```python
from build123d import *

# Parameters (mm, degrees)
PAD_DEPTH       = 50
POCKET_DEPTH    = 50.001
FILLET_R        = 0.5
SKETCH003_R     = 7.438429
POCKET001_DEPTH = 24.66558


with BuildPart() as part:
    # Sketch → Pad (new body)
    with BuildSketch(Plane.XY):
        with BuildLine():
            Line((0, 15), (0, 0))
            Line((0, 0), (50, 0))
            Line((50, 0), (50, 20))
            ThreePointArc((50, 20), (47.363119, 25.733162), (41.294118, 27.462185))
            Line((41.294118, 27.462185), (6, 22))
            ThreePointArc((6, 22), (1.705266, 19.609772), (0, 15))
        make_face()
    extrude(amount=PAD_DEPTH)

    # Sketch002 → Pocket (cut, through all)
    with BuildSketch(Plane.XY):
        with BuildLine():
            Line((1.617649, 14.859023), (1.617649, 2.886441))
            Line((1.617649, 2.886441), (48.358659, 2.886441))
            Line((48.358659, 2.886441), (48.358659, 20.203976))
            ThreePointArc((48.358659, 20.203976), (46.261778, 24.757846), (41.4384, 26.125203))
            Line((41.4384, 26.125203), (6.589663, 20.669917))
            ThreePointArc((6.589663, 20.669917), (3.030296, 18.682876), (1.617649, 14.859023))
        make_face()
    extrude(amount=POCKET_DEPTH, mode=Mode.SUBTRACT)

    # Fillet
    fillet_edges = [part.edges().sort_by_distance(p)[0] for p in [
        (25, 0, 50),
        (0, 7.5, 50),
        (1.705266, 19.609772, 50),
        (23.647059, 24.731092, 50),
        (47.363119, 25.733162, 50),
        (50, 10, 50),
        (50, 10, 0),
        (25, 0, 0),
        (50, 0, 25),
        (0, 0, 25),
    ]]
    fillet(fillet_edges, radius=FILLET_R)

    # Sketch003 (on Face21 of Fillet) → Pocket001 (cut, through all)
    with BuildSketch(Plane(origin=(0, 2.886441, 0), x_dir=(-1, 0, 0), z_dir=(0, 1, 0))):
        with Locations((-24.985147, 24.818342)):
            Circle(SKETCH003_R)
    extrude(amount=POCKET001_DEPTH, mode=Mode.SUBTRACT)


solid = part.part
```
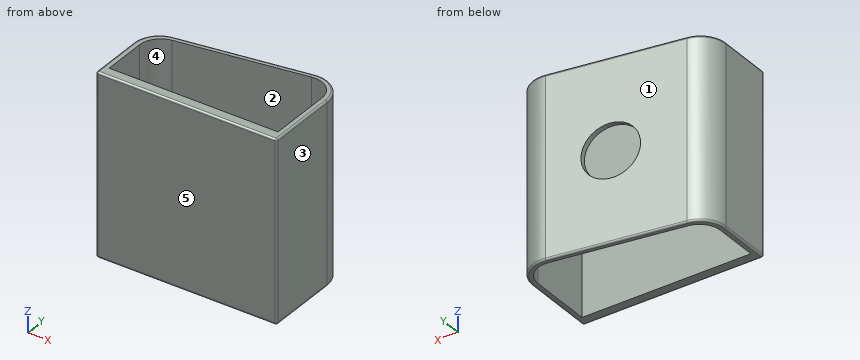
Can you work these out from the model? Positions are in its coordinate system, mm. Face numbers are marked on the shaded views. A direction names the side the tool comes from. Round coordinates to 2 decimals unless told otherwise and drop trailing zeros. Loops run counter-clockwise (first coordinate to the right, second up) from the corner with the lowest first, then second, coordinate; pieces in that order, holes last. Notation, with made-up numbers: M 3.25,7 L 38.25,7 A16 ccw 38.25,37 Z; hole C 29.25,-15 d4. An arc over 180 degrees is marked long. Answer in a Markdown table with one row per item.
1. If we section it at A-A, the plane y = 13.75: Please give me the cut outline in (x, z), plus the area to 3 significant figures.
Established:
| item | result |
|---|---|
| outline | M 0,0.5 A0.5 ccw 0.5,0 L 1.62,0 L 1.62,50 L 0.5,50 A0.5 ccw 0,49.5 Z; M 48.36,0 L 49.5,0 A0.5 ccw 50,0.5 L 50,49.5 A0.5 ccw 49.5,50 L 48.36,50 Z |
| area | 163 mm² |
2. If we section it at D-D, the plane x = 28: Give the number of separate pieces and of enclosed holes in the cut face, plus the area to 3 significant figures.
Established:
| item | result |
|---|---|
| separate pieces | 3 |
| enclosed holes | 0 |
| area | 194 mm² |
3. If we section it at C-C, the plane z = 27: Please give me the cut outline in (x, y).
Established:
| item | result |
|---|---|
| outline | M 0,0.5 A0.5 ccw 0.5,0 L 49.5,0 A0.5 ccw 50,0.5 L 50,20 A7.55 ccw 41.29,27.46 L 32.1,26.04 L 32.1,24.66 L 41.44,26.13 A5.99 cw 48.36,20.2 L 48.36,2.89 L 1.62,2.89 L 1.62,14.86 A5.88 cw 6.59,20.67 L 17.87,22.44 L 17.87,23.84 L 6,22 A7.08 ccw 0,15 Z |
4. On a 3-axis mill with a long thin cutter (end or side, diameter ignored), from which of +Z, -Z, +X, -X, +Y, -Y can I reach the whole of each face in a straight line? I mean the marked faces 4 and 5. Say none if no direction works.
Established:
| item | result |
|---|---|
| face 4 | +Z, -Z |
| face 5 | +Z, -Z, +X, -X, -Y |
5. Please list where these lines run through material, in increasing order: line 1 (X direction, y = 12.5, z = 34); line 2 (Y direction, x = 26.5, z = 29.5); line 3 (Y direction, x = 32, z = 19). Write a range as from..to.
Established:
| item | result |
|---|---|
| line 1 | 0..1.62, 48.36..50 |
| line 2 | 0..2.89 |
| line 3 | 0..2.89, 24.65..26.02 |
6. I'm going to push flat-ended pins straight in: pin 1 Ø5 at (x, z) = (18, 25.5) entering from +Y; pin 2 Ø10 at (x, y) = (20.5, 18.5) entering from +Z; pin 3 Ø1 at (x, z) = (7, 44) entering from +Y. Where does each tip first touch, or does it pass through?
Established:
| item | result |
|---|---|
| pin 1 | y = 23.9 |
| pin 2 | z = 50 |
| pin 3 | y = 22.23 |
7. If we section it at B-B, the plane z = 9: Please give me the cut outline in (x, y), plus the area to 3 significant figures.
Established:
| item | result |
|---|---|
| outline | M 0,0.5 A0.5 ccw 0.5,0 L 49.5,0 A0.5 ccw 50,0.5 L 50,20 A7.55 ccw 41.29,27.46 L 6,22 A7.08 ccw 0,15 Z; hole M 1.62,2.89 L 48.36,2.89 L 48.36,20.2 A5.99 ccw 41.44,26.13 L 6.59,20.67 A5.88 ccw 1.62,14.86 Z |
| area | 272 mm² |
8. Thinking about a two-plate mould opening in Y: for the marked faces 1, 2 and 3, which applies, pulls with the +Y half, pulls with the -Y half, needs draft (parallel to the pull), parting line crosses it, or undercut?
Established:
| item | result |
|---|---|
| face 1 | pulls with the +Y half |
| face 2 | undercut |
| face 3 | needs draft |
